Build history of the part. All positions in model axes, mm. Face numbers are marked on the shaded views. A direction names the side the tool comes from. Give positions to 0.01 mm unless a question says otherwise; leave off trailing zeros. Loops run counter-clockwise (first coordinate to the right, second up) from the corner with the lowest first, then second, coordinate; pieces in that order, holes last.
1) Wall check: line 1 (Z direction, x = 9.25, y = 6.75); line 2 (X direction, y = 9.75, z = -9); line 3 (Y direction, x = 10.25, z = -3.5). Give the ranges that are in metal, low to high.
2) Band-saw the part on A-A on z = 0. List the corners of the cut face in (x, y), then the cut area to 3 significant figures.
3) Band-saw the part on D-D on z = -7.75. List the corners of the cut face in (x, y).
4) Band-saw the part on B-B on y = 6. List the corners of the cut face in (x, z).
5) Flat gauge pins, fed straight in: P1, Ø1, axis at x = 8, y = 10.5, coming from the +Z side; P2, Ø0.9, axis at x = -11, z = -4, coming from the -Y side; P3, Ø3, axis at x = 6, z = 0, coming from the +Y side; P4, Ø1.5, axis at y = -11, z = -2.5, coming from the -X side. Where does each tip first touch, or does it go through?
6) 3-axis set-ups, long thin cutter, end or side, ignore diameter. For the marked faces 1, 2 and 3: which of +Z, -Z, +X, -X, +Y, -Y reach the whole face in a straight line?
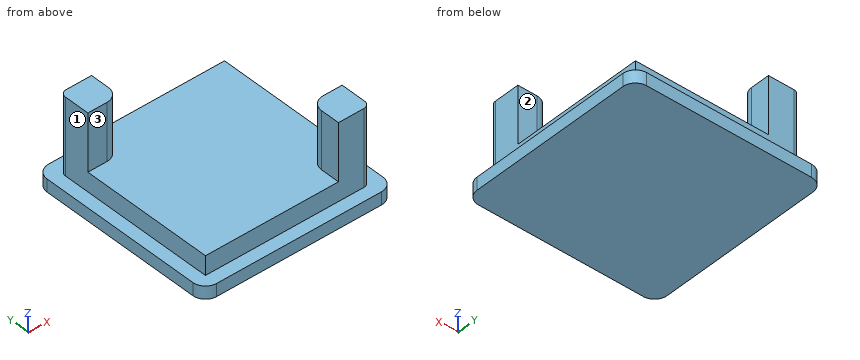
```python
from build123d import *

# Parameters (mm, degrees)
BOX013_W     = 26
BOX013_H     = 26
BOX013_DEPTH = 3
BOX014_W     = 5
BOX014_H     = 5
BOX014_DEPTH = 9
BOX012_W     = 30
BOX012_H     = 30
BOX012_DEPTH = 2
BOX015_W     = 5
BOX015_H     = 5
BOX015_DEPTH = 9
FILLET001_R  = 2
FILLET002_R  = 2
FILLET003_R  = 1


with BuildPart() as obj1:
    # Box013 → Box013 (new body)
    with BuildSketch(Plane(origin=(-13, -13, -10), x_dir=(1, 0, 0), z_dir=(0, 0, 1))):
        with Locations((13, 13)):
            Rectangle(BOX013_W, BOX013_H)
    extrude(amount=BOX013_DEPTH)


with BuildPart() as obj2:
    # Box014 → Box014 (new body)
    with BuildSketch(Plane(origin=(-13, 8, -7), x_dir=(1, 0, 0), z_dir=(0, 0, 1))):
        with Locations((2.5, 2.5)):
            Rectangle(BOX014_W, BOX014_H)
    extrude(amount=BOX014_DEPTH)


with BuildPart() as obj3:
    # Box012 → Box012 (new body)
    with BuildSketch(Plane(origin=(-15, -15, -12), x_dir=(1, 0, 0), z_dir=(0, 0, 1))):
        with Locations((15, 15)):
            Rectangle(BOX012_W, BOX012_H)
    extrude(amount=BOX012_DEPTH)


with BuildPart() as fillet003:
    # Box015 → Box015 (new body)
    with BuildSketch(Plane(origin=(8, -13, -7), x_dir=(1, 0, 0), z_dir=(0, 0, 1))):
        with Locations((2.5, 2.5)):
            Rectangle(BOX015_W, BOX015_H)
    extrude(amount=BOX015_DEPTH)

    # Fusion004: union obj1, obj2, obj3
    add(obj1.part)
    add(obj2.part)
    add(obj3.part)

    # Fillet001
    fillet001_edges = [fillet003.edges().sort_by_distance(p)[0] for p in [
        (-15, -15, -11),
        (-15, 15, -11),
        (15, 15, -11),
        (15, -15, -11),
    ]]
    fillet(fillet001_edges, radius=FILLET001_R)

    # Fillet002
    fillet002_edges = [fillet003.edges().sort_by_distance(p)[0] for p in [
        (-8, 8, -2.5),
        (8, -8, -2.5),
    ]]
    fillet(fillet002_edges, radius=FILLET002_R)

    # Fillet003
    fillet003_edges = [fillet003.edges().sort_by_distance(p)[0] for p in [
        (-13, 13, -2.5),
        (13, -13, -2.5),
    ]]
    fillet(fillet003_edges, radius=FILLET003_R)


solid = fillet003.part
```
Findings below:
1. line 1: z = -12 to -7
1. line 2: x = -13 to 13
1. line 3: y = -13 to -8
2. outline: (-13, 8) - (-10, 8) arc R2 ccw to (-8, 10) - (-8, 13) - (-12, 13) arc R1 ccw to (-13, 12) - close; (8, -13) - (12, -13) arc R1 ccw to (13, -12) - (13, -8) - (10, -8) arc R2 ccw to (8, -10) - close
2. area: 47.9 mm2
3. outline: (-13, -13) - (12, -13) arc R1 ccw to (13, -12) - (13, 13) - (-12, 13) arc R1 ccw to (-13, 12) - close
4. outline: (-15, -12) - (15, -12) - (15, -10) - (13, -10) - (13, -7) - (-13, -7) - (-13, -10) - (-15, -10) - close
5. P1: stops at z = -7
5. P2: stops at y = 8
5. P3: passes through
5. P4: stops at x = 8
6. face 1: +Z, -X, +Y, -Y
6. face 2: +Z, +X, -X, +Y
6. face 3: +Z, +X, -X, -Y
